For this review, take the finished solid that the model builds, in its own axes (mm). Face numbers are marked on the shaded views. A direction names the side the tool comes from. Coordinates: 2 decimals unless noted, no trailing zeros. Write each loop counter-clockwise with the first axis right and the second up, starting at its lowest first coordinate (ties: lowest second). Pieces come first, ordered by that corner, then holes. Notation, with made-up numbers: (35.25, -32.5) -> (92.25, -32.5) arc R22 ccw to (92.25, -1.5) -> close; hole circle Ø6 at (34, 42). An arc over 180 degrees is marked (long way). Put each result on its own line as item: value. Start each with the question number.
Item 1: Consider section B-B on y = 0. Give the boundary of the cut face in (x, z) (3 decimals).
Item 2: For the marked faces 1 and 2, list the 3-axis set-ups (+Z, -Z, +X, -X, +Y, -Y) from which the entire face can be reached by the end or side of a thin tool; tool diameter is ignored.
Item 3: Consider section D-D on x = -5.25. Give the boundary of the cut face in (y, z), and give its area (3 significant figures).
Item 4: To check wall thickness, follow L1, parallel to Z at x = 1.25, y = -0.05 (3 decimals); L2, parallel to X at y = -1.8, z = -0.75; L3, parallel to Z at x = -0.75, y = -0.8. State the ranges of each line that lie inside material, in increasing order.
Item 5: Insertion check: P1, Ø2, axis at x = 3, y = -1.5, coming from the +Z side. The pin has a flat end and moves straight along its axis. Give the tip position at first contact, or say it passes through.
Item 6: Consider section C-C on x = 3.5. Give the boundary of the cut face in (y, z) (3 decimals).
Item 7: The part is to be moulded in two halves that separate along X. For the marked faces 3, 4 and 5, say which applies: +X half, -X half, draft (parallel to the pull), parting line (faces both ways), or undercut.
Item 8: Consider section A-A on z = 0. Give the boundary of the cut face in (x, y).
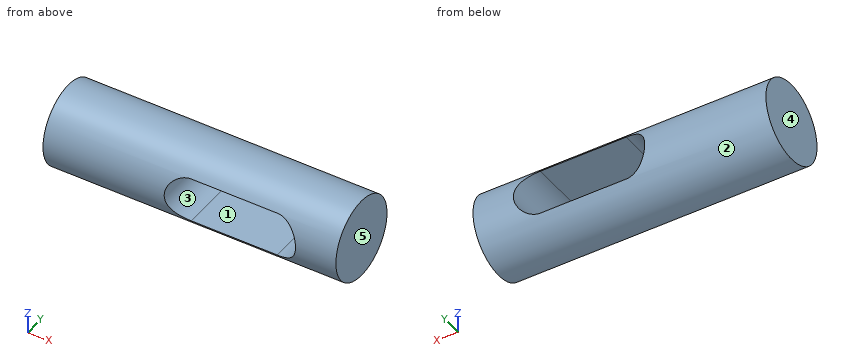
```python
from build123d import *

# Parameters (mm, degrees)
SKETCH1_W               = 14.5
SKETCH1_H               = 2
CUT_EXTRUDE1_DEPTH      = 8.782191208
CUT_EXTRUDE1_DEPTH_BACK = 8.782191208


with BuildPart() as part:
    # Sketch1 → Revolve1 (revolve)
    with BuildSketch(Plane(origin=(0, 0, 0), x_dir=(1, 0, 0), z_dir=(0, 1, 0)), mode=Mode.PRIVATE) as revolve1_sk:
        with Locations((0, 1)):
            Rectangle(SKETCH1_W, SKETCH1_H)
    revolve(revolve1_sk.sketch.rotate(Axis((-7.25, 0, 0), (1, 0, 0)), 180), axis=Axis((-7.25, 0, 0), (1, 0, 0)))

    # Sketch2 → Cut-Extrude1 (cut, two sides: drawn at the far end of the back side and taken through both)
    with BuildSketch(Plane(origin=(0, 0, 0), x_dir=(1, 0, 0), z_dir=(0, 1, 0)).offset(-CUT_EXTRUDE1_DEPTH_BACK)):
        with BuildLine():
            Line((-0.125, 1.125), (4.125, 1.125))
            ThreePointArc((4.125, 1.125), (5.25, 0), (4.125, -1.125))
            Line((4.125, -1.125), (-0.125, -1.125))
            ThreePointArc((-0.125, -1.125), (-1.25, 0), (-0.125, 1.125))
        make_face()
    extrude(amount=CUT_EXTRUDE1_DEPTH + CUT_EXTRUDE1_DEPTH_BACK, mode=Mode.SUBTRACT)


solid = part.part
```
Return value:
1. outline: (-7.25, -2) -> (7.25, -2) -> (7.25, 2) -> (-7.25, 2) -> close; hole (-0.125, -1.125) -> (4.125, -1.125) arc R1.125 ccw to (4.125, 1.125) -> (-0.125, 1.125) arc R1.125 ccw to start
2. face 1: +Y, -Y
2. face 2: +X, -X
3. outline: circle Ø4 at (0, 0)
3. area: 12.6 mm^2
4. L1: -1.999 to -1.125, 1.125 to 1.999
4. L2: -7.25 to -0.96, 4.96 to 7.25
4. L3: -1.83 to -0.94, 0.94 to 1.83
5. P1: z = 1.94
6. outline: (-1.654, -1.125) arc R2 ccw to (1.654, -1.125) -> close; (-1.654, 1.125) -> (1.654, 1.125) arc R2 ccw to start
7. face 3: undercut
7. face 4: -X half
7. face 5: +X half
8. outline: (-7.25, -2) -> (-1.25, -2) -> (-1.25, 2) -> (-7.25, 2) -> close; (5.25, -2) -> (7.25, -2) -> (7.25, 2) -> (5.25, 2) -> close
